Can you work these out from the model? Positions are in its coordinate system, mm. A direction names the side the tool comes from. Round coordinates to 2 decimals unless told otherwise and drop trailing zeros. Loops run counter-clockwise (first coordinate to the right, second up) from the corner with the lowest first, then second, coordinate; pieces in that order, holes last. Notation, with made-up numbers: (15.25, -15) -> (30.25, -15) arc R24 cw to (30.25, 7) -> close; hole circle Ø2 at (48, 60.5). An arc over 180 degrees is marked (long way). Write item = value, one per line.
from build123d import *

# Parameters (mm, degrees)
SKETCH_1_W          = 16
SKETCH_1_H          = 21
SKETCH_1_R          = 1.75
EXTRUDE_1_DEPTH     = 5
EXTRUDE_1_2_DEPTH   = 16
CUT_EXTRUDE_1_DEPTH = 16
SKETCH_4_W          = 3.81913455
SKETCH_4_H          = 4
CUT_EXTRUDE_2_DEPTH = 2.5
SKETCH_5_R          = 0.1
CUT_EXTRUDE_3_DEPTH = 2
SKETCH_6_W          = 6.153050109
SKETCH_6_H          = 6.032352941
CUT_EXTRUDE_4_DEPTH = 10


with BuildPart() as part:
    # Эскиз1 → Extrude 1 (new body)
    with BuildSketch(Plane.XY):
        with Locations((0, 5)):
            Rectangle(SKETCH_1_W, SKETCH_1_H)
        Circle(SKETCH_1_R, mode=Mode.SUBTRACT)
    extrude(amount=EXTRUDE_1_DEPTH)

    # Эскиз2 → Extrude 1 2 (add)
    with BuildSketch(Plane.ZY.offset(8)):
        with BuildLine():
            Line((2.675, 15.5), (2.675, 19))
            ThreePointArc((2.675, 19), (2.916636906, 19.583363094), (3.5, 19.825))
            Line((3.5, 19.825), (11, 19.825))
            Line((11, 19.825), (11, 20.175))
            Line((11, 20.175), (3.5, 20.175))
            ThreePointArc((3.5, 20.175), (2.669149532, 19.830850468), (2.325, 19))
            Line((2.325, 19), (2.325, 15.5))
            Line((2.325, 15.5), (2.675, 15.5))
        make_face()
    extrude(amount=-EXTRUDE_1_2_DEPTH)

    # Эскиз3 → Вырез-Вытянуть1 (cut)
    with BuildSketch(Plane(origin=(0, 0, 2.325), x_dir=(-1, 0, 0), z_dir=(0, 0, -1))):
        Polygon((-1.75, 15.5), (-1.75, 18.5), (-0.55, 19), (-0.55, 20.937907948), (-4.95, 20.937907948), (-4.95, 19), (-4.4, 18.622085888), (-4.4, 15.5), align=None)
        Polygon((0.55, 19), (0.55, 20.937907948), (4.95, 20.937907948), (4.95, 19), (4.4, 18.622085888), (4.4, 15.5), (1.75, 15.5), (1.75, 18.5), align=None)
        Polygon((-6.05, 19), (-6.05, 20.937907948), (-9.320905805, 20.937907948), (-9.320905805, 15.5), (-6.6, 15.5), (-6.6, 18.622085888), align=None)
        Polygon((6.05, 19), (6.05, 20.937907948), (9.499807758, 20.937907948), (9.499807758, 15.5), (6.6, 15.5), (6.6, 18.622085888), align=None)
    extrude(amount=-CUT_EXTRUDE_1_DEPTH, mode=Mode.SUBTRACT)

    # Эскиз4 → Вырез-Вытянуть2 (cut)
    with BuildSketch(Plane(origin=(0, 0, 5), x_dir=(-1, 0, 0), z_dir=(0, 0, -1))):
        with Locations((7.909567275, 0)):
            Rectangle(SKETCH_4_W, SKETCH_4_H)
        with Locations((-7.909567275, 0)):
            Rectangle(SKETCH_4_W, SKETCH_4_H)
    extrude(amount=CUT_EXTRUDE_2_DEPTH, mode=Mode.SUBTRACT)

    # Эскиз5 → Вырез-Вытянуть3 (cut)
    with BuildSketch(Plane.XY.offset(11)):
        with Locations((-5.45, 20)):
            Circle(SKETCH_5_R)
    extrude(amount=-CUT_EXTRUDE_3_DEPTH, mode=Mode.SUBTRACT)

    # Эскиз6 → Вырез-Вытянуть4 (cut)
    with BuildSketch(Plane(origin=(0, 0, 2.325), x_dir=(-1, 0, 0), z_dir=(0, 0, -1))):
        with Locations((0.350490197, 18.516176471)):
            Rectangle(SKETCH_6_W, SKETCH_6_H)
    extrude(amount=-CUT_EXTRUDE_4_DEPTH, mode=Mode.SUBTRACT)


solid = part.part
1. I need wall thicknesses on line 1 (X direction, y = 20, z = 10.1); line 2 (Z direction, x = -2.5, y = 1.75); line 3 (Y direction, x = 0, z = 2.55). Which ranges of each line are inside material? Lowest first, please. Write a range as [from, to].
Entries:
line_1 = [-6.05, -5.55], [-5.35, -4.95], [4.95, 6.05]
line_2 = [0, 5]
line_3 = [-5.5, -1.75], [1.75, 15.5]
2. Suppose I cut it at D-D, the plane z = 5.5. List the corners of the cut face in (x, y) for me (3 decimals), and give its area (3 significant figures).
Entries:
outline = (-6.05, 19.825) -> (-4.95, 19.825) -> (-4.95, 20.175) -> (-6.05, 20.175) -> close; (4.95, 19.825) -> (6.05, 19.825) -> (6.05, 20.175) -> (4.95, 20.175) -> close
area = 0.770 mm²
3. We'd pull the mould along X, two halves only. Please class faces 1 (the flat face through (-7, 0, 2.5)), 2 (the flat face through (-8, 5, 2)), 3 (the cylindrical face through (1.617, -0.67, 2.465)): released by +X, released by -X, zero draft, split by the parting line, or undercut.
Entries:
face_1 = zero draft
face_2 = released by -X
face_3 = undercut
4. For faces 4 (the flat face through (5.5, 20.175, 7.3)), 5 (the flat face through (-5.5, 19.825, 7.2)), 6 (the flat face through (-7, 2, 4)), 7 (the flat face through (0, 5, 5)), 8 (the flat face through (7, -2, 4)), which set-ups out of +Z, -Z, +X, -X, +Y, -Y let a thin tool reach every point of the face, with its end or its side?
Entries:
face_4 = +Z, -Z, +X, -X, +Y
face_5 = +Z, +X, -X
face_6 = +Z, -X
face_7 = +Z, +X, -X, -Y
face_8 = +Z, +X
5. Suppose I cut it at B-B, the plane x = 0. List the corners of the cut face in (y, z) for me.
Entries:
outline = (-5.5, 0) -> (-1.75, 0) -> (-1.75, 5) -> (-5.5, 5) -> close; (1.75, 0) -> (15.5, 0) -> (15.5, 5) -> (1.75, 5) -> close
6. Suppose I cut it at A-A, the plane z = 10.25. List the corners of the cut face in (x, y) for me (3 decimals).
Entries:
outline = (-6.05, 19.825) -> (-4.95, 19.825) -> (-4.95, 20.175) -> (-6.05, 20.175) -> close; (4.95, 19.825) -> (6.05, 19.825) -> (6.05, 20.175) -> (4.95, 20.175) -> close; hole circle Ø0.2 at (-5.45, 20)
7. Suppose I cut it at C-C, the plane y = 0. List the corners of the cut face in (x, z) for me, and give its area (3 significant figures).
Entries:
outline = (-8, 0) -> (-1.75, 0) -> (-1.75, 5) -> (-6, 5) -> (-6, 2.5) -> (-8, 2.5) -> close; (1.75, 0) -> (8, 0) -> (8, 2.5) -> (6, 2.5) -> (6, 5) -> (1.75, 5) -> close
area = 52.5 mm²
8. I'm going to push flat-ended pins straight in: pin 1 (4 mm diameter, centred on x = 4.5, y = 16, fed in from +Z); pin 2 (0.9 mm diameter, centred on y = 19.5, z = 7.5, fed in from +X); pin 3 (1.1 mm diameter, centred on x = -5.5, y = 16.5, fed in from -Z) (3 decimals). Where does each tip first touch, or does it pass through?
Entries:
pin_1 = 5
pin_2 = 6.05
pin_3 = 2.325
